Geometry check sheet. Reference: the model listing, model coordinates, mm. A direction names the side the tool comes from. Round coordinates to 2 decimals unless told otherwise and drop trailing zeros. Order: outer loops, then holes, each group sorted by start corner. A loop starts at its lowest first (then second) coordinate and runs counter-clockwise, first axis right, second up. Notation, with made-up numbers: (78.25, -12) - (117.25, -12) arc R30 cw to (117.25, 17) - close; hole circle Ø1 at (-3.75, -3). An arc over 180 degrees is marked (long way). Use a Markdown table: item, result. Add a question column.
(1) Thickness scan on line 1 along X through (y, z) = (1, -4.25); line 2 along Y through (x, z) = (-1, -3); line 3 along Z through (x, y) = (-4.75, 6). Record the ranges inside material, lowest first. Write a range as [from, to].
(2) Access from +Z, -Z, +X, -X, +Y, -Y to the whole of each face (thin tool, end or side, straight path). Record for faces 1 (the face through (-4.573, 5, 1)), 2 (the face through (0, -6, -5)), 3 (the face through (0, 7.65, -2)).
(3) Section check C-C on z = -0.75. Record the boundary of the cut face in (x, y).
(4) Section check B-B on z = 1. Record the boundary of the cut face in (x, y).
(5) Mould release check, pull along X, two halves, no side actions. Record for faces 4 (the face through (5.227, 5, 1)), 5 (the face through (8.877, 1, -1)), 6 (the face through (0, 10.1, -1)), 7 (the face through (6.427, 2, -2)): released by +X, released by -X, zero draft, split by the parting line, or undercut.
(6) Gauge pin test, flat end, axial feed: P1, Ø10, axis at x = 3.5, y = 3.5, coming from the -Z side. Record the tip position at first contact, or that the pin passes through.
(7) Section check D-D on x = 2.75. Record the boundary of the cut face in (y, z).
(8) Section check A-A on x = -3.75. Record the boundary of the cut face in (y, z).
```python
from build123d import *

# Parameters (mm, degrees)
F1_DEPTH = 5
F2_DEPTH = 2.4


with BuildPart() as f1:
    # F0 (on Top) → F1 (new body)
    with BuildSketch(Plane.XY):
        with BuildLine():
            Line((-8.2229121849, -7), (8.8770878151, -7))
            Line((8.8770878151, -7), (8.8770878151, -4.5))
            Line((8.8770878151, -4.5), (8.8770878151, 1.55))
            Line((8.8770878151, 1.55), (6.4270878151, 1.55))
            Line((6.4270878151, 1.55), (6.4270878151, -4.55))
            Line((6.4270878151, -4.55), (3.9714117296, -4.55))
            ThreePointArc((3.9714117296, -4.55), (1.0867994279, -5.4234526619), (-1.7978128738, -4.55))
            Line((-1.7978128738, -4.55), (-5.7729121849, -4.55))
            Line((-5.7729121849, -4.55), (-5.7729121849, 1.55))
            Line((-5.7729121849, 1.55), (-8.2229121849, 1.55))
            Line((-8.2229121849, 1.55), (-8.2229121849, -7))
        make_face()
        Polygon((-8.2229121849, 10.1), (-8.2229121849, 1.55), (-5.7729121849, 1.55), (-5.7729121849, 7.65), (6.4270878151, 7.65), (6.4270878151, 1.55), (8.8770878151, 1.55), (8.8770878151, 7.6), (8.8770878151, 10.1), align=None)
        with BuildLine():
            Line((3.9714117296, -4.55), (-1.7978128738, -4.55))
            ThreePointArc((-1.7978128738, -4.55), (1.0867994279, -5.4234526619), (3.9714117296, -4.55))
        make_face()
    extrude(amount=-F1_DEPTH)

    # F0 (on Top) → F2 (join)
    with BuildSketch(Plane.XY):
        Polygon((-8.2229121849, 10.1), (-8.2229121849, 1.55), (-5.7729121849, 1.55), (-5.7729121849, 7.65), (6.4270878151, 7.65), (6.4270878151, 1.55), (8.8770878151, 1.55), (8.8770878151, 7.6), (8.8770878151, 10.1), align=None)
        with BuildLine():
            Line((-5.7729121849, 7.65), (-5.7729121849, 1.55))
            Line((-5.7729121849, 1.55), (-3.8014380516, 1.55))
            ThreePointArc((-3.8014380516, 1.55), (-2.776349623, 3.2573632497), (-1.1846618734, 4.4542031139))
            Line((-1.1846618734, 4.4542031139), (-4.5729121849, 4.4542031139))
            Line((-4.5729121849, 4.4542031139), (-4.5729121849, 6.4542031139))
            Line((-4.5729121849, 6.4542031139), (5.2270878151, 6.4542031139))
            Line((5.2270878151, 6.4542031139), (5.2270878151, 4.4542031139))
            Line((5.2270878151, 4.4542031139), (3.3582607291, 4.4542031139))
            ThreePointArc((3.3582607291, 4.4542031139), (4.9499484788, 3.2573632497), (5.9750369074, 1.55))
            Line((5.9750369074, 1.55), (6.4270878151, 1.55))
            Line((6.4270878151, 1.55), (6.4270878151, 7.65))
            Line((6.4270878151, 7.65), (-5.7729121849, 7.65))
        make_face()
        with BuildLine():
            ThreePointArc((-1.1846618734, 4.4542031139), (-2.776349623, 3.2573632497), (-3.8014380516, 1.55))
            Line((-3.8014380516, 1.55), (-1.3328835382, 1.55))
            ThreePointArc((-1.3328835382, 1.55), (-0.6001096537, 2.2573411124), (0.3270878151, 2.678759988))
            Line((0.3270878151, 2.678759988), (0.3270878151, 4.4542031139))
            Line((0.3270878151, 4.4542031139), (-1.1846618734, 4.4542031139))
        make_face()
        with BuildLine():
            Line((3.5064823939, 1.55), (5.9750369074, 1.55))
            ThreePointArc((5.9750369074, 1.55), (4.9499484788, 3.2573632497), (3.3582607291, 4.4542031139))
            Line((3.3582607291, 4.4542031139), (0.3270878151, 4.4542031139))
            Line((0.3270878151, 4.4542031139), (0.3270878151, 2.678759988))
            ThreePointArc((0.3270878151, 2.678759988), (2.0904931068, 2.6036658356), (3.5064823939, 1.55))
        make_face()
        with BuildLine():
            Line((-1.3328835382, 1.55), (-3.8014380516, 1.55))
            ThreePointArc((-3.8014380516, 1.55), (-3.8535242893, -1.8461669219), (-1.7978128738, -4.55))
            Line((-1.7978128738, -4.55), (3.9714117296, -4.55))
            ThreePointArc((3.9714117296, -4.55), (5.6715559082, -2.6770231246), (6.2867994279, -0.2234526619))
            ThreePointArc((6.2867994279, -0.2234526619), (6.2082657654, 0.6768709207), (5.9750369074, 1.55))
            Line((5.9750369074, 1.55), (3.5064823939, 1.55))
            ThreePointArc((3.5064823939, 1.55), (3.938031521, 0.7095401307), (4.0867994279, -0.2234526619))
            ThreePointArc((4.0867994279, -0.2234526619), (0.1538066353, -3.074684755), (-1.3328835382, 1.55))
        make_face()
        with BuildLine():
            Line((-3.8014380516, 1.55), (-5.7729121849, 1.55))
            Line((-5.7729121849, 1.55), (-5.7729121849, -4.55))
            Line((-5.7729121849, -4.55), (-1.7978128738, -4.55))
            ThreePointArc((-1.7978128738, -4.55), (-3.8535242893, -1.8461669219), (-3.8014380516, 1.55))
        make_face()
        with BuildLine():
            Line((-8.2229121849, -7), (8.8770878151, -7))
            Line((8.8770878151, -7), (8.8770878151, -4.5))
            Line((8.8770878151, -4.5), (8.8770878151, 1.55))
            Line((8.8770878151, 1.55), (6.4270878151, 1.55))
            Line((6.4270878151, 1.55), (6.4270878151, -4.55))
            Line((6.4270878151, -4.55), (3.9714117296, -4.55))
            ThreePointArc((3.9714117296, -4.55), (1.0867994279, -5.4234526619), (-1.7978128738, -4.55))
            Line((-1.7978128738, -4.55), (-5.7729121849, -4.55))
            Line((-5.7729121849, -4.55), (-5.7729121849, 1.55))
            Line((-5.7729121849, 1.55), (-8.2229121849, 1.55))
            Line((-8.2229121849, 1.55), (-8.2229121849, -7))
        make_face()
        with BuildLine():
            Line((3.9714117296, -4.55), (-1.7978128738, -4.55))
            ThreePointArc((-1.7978128738, -4.55), (1.0867994279, -5.4234526619), (3.9714117296, -4.55))
        make_face()
        with BuildLine():
            Line((6.4270878151, -4.55), (6.4270878151, 1.55))
            Line((6.4270878151, 1.55), (5.9750369074, 1.55))
            ThreePointArc((5.9750369074, 1.55), (6.2082657654, 0.6768709207), (6.2867994279, -0.2234526619))
            ThreePointArc((6.2867994279, -0.2234526619), (5.6715559082, -2.6770231246), (3.9714117296, -4.55))
            Line((3.9714117296, -4.55), (6.4270878151, -4.55))
        make_face()
    extrude(amount=F2_DEPTH)


solid = f1.part
```
Check sheet entries:
| question | item | result |
|---|---|---|
| 1 | line 1 | x = [-8.22, -5.77], [6.43, 8.88] |
| 1 | line 2 | y = [-7, -4.55], [7.65, 10.1] |
| 1 | line 3 | z = [0, 2.4] |
| 2 | face 1 | +Z, -Z |
| 2 | face 2 | -Z, +X, -X, +Y, -Y |
| 2 | face 3 | -Z |
| 3 | outline | (-8.22, -7) - (8.88, -7) - (8.88, 10.1) - (-8.22, 10.1) - close; hole (-5.77, -4.55) - (6.43, -4.55) - (6.43, 7.65) - (-5.77, 7.65) - close |
| 4 | outline | (-8.22, -7) - (8.88, -7) - (8.88, 10.1) - (-8.22, 10.1) - close; hole (-4.57, 4.45) - (5.23, 4.45) - (5.23, 6.45) - (-4.57, 6.45) - close; hole circle Ø6 at (1.09, -0.22) |
| 5 | face 4 | undercut |
| 5 | face 5 | released by +X |
| 5 | face 6 | zero draft |
| 5 | face 7 | undercut |
| 6 | P1 | stops at z = -5 |
| 7 | outline | (-7, -5) - (-4.55, -5) - (-4.55, 0) - (-2.72, 0) - (-2.72, 2.4) - (-7, 2.4) - close; (2.27, 0) - (4.45, 0) - (4.45, 2.4) - (2.27, 2.4) - close; (6.45, 0) - (7.65, 0) - (7.65, -5) - (10.1, -5) - (10.1, 2.4) - (6.45, 2.4) - close |
| 8 | outline | (-7, -5) - (-4.55, -5) - (-4.55, 0) - (4.45, 0) - (4.45, 2.4) - (-7, 2.4) - close; (6.45, 0) - (7.65, 0) - (7.65, -5) - (10.1, -5) - (10.1, 2.4) - (6.45, 2.4) - close |
